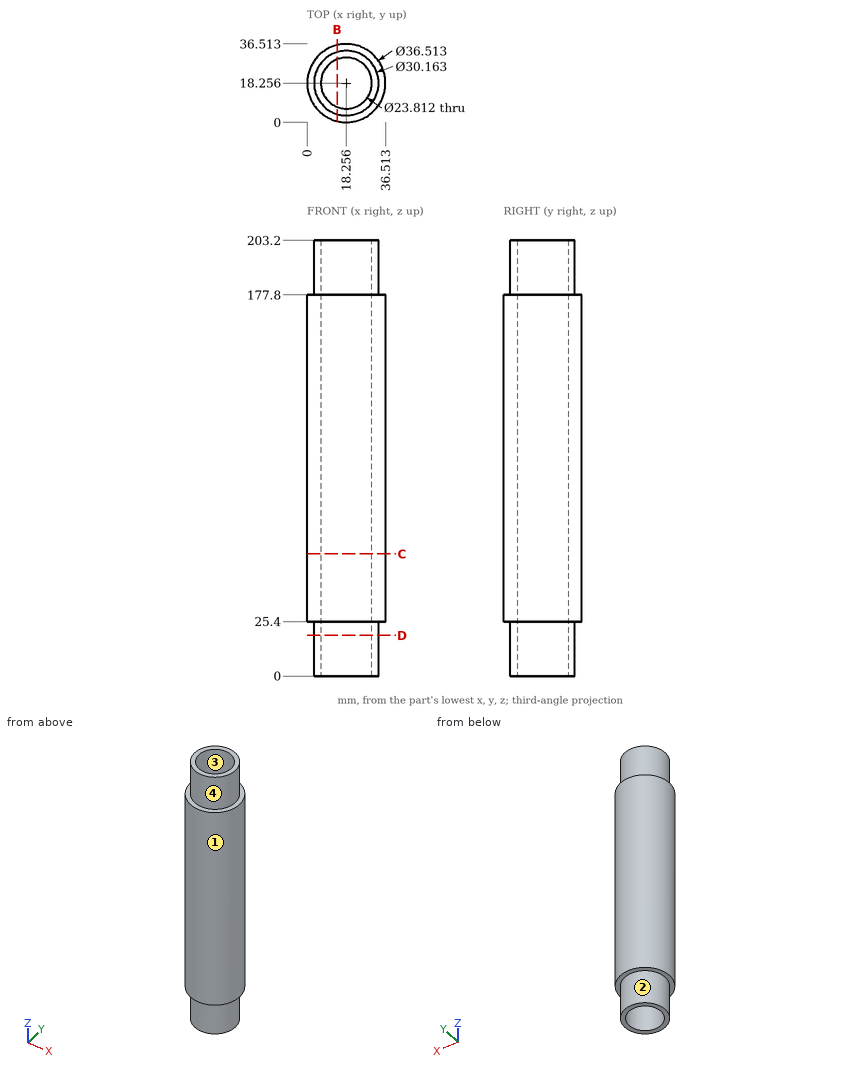
For this review, use the dimensioned drawing (mm, ordinates from the lowest corner) and the shaded views. A direction names the side the tool comes from. Round coordinates to 2 decimals unless told otherwise and drop trailing zeros. Write each loop counter-clockwise with the first axis right and the second up, starting at its lowest first coordinate (ties: lowest second). Pieces come first, ordered by that corner, then holes. Notation, with made-up numbers: (65.25, 21.25) -> (121.25, 21.25) arc R29 ccw to (121.25, 57.25) -> close; hole circle Ø11 at (56, 70.25). An arc over 180 degrees is marked (long way). Use one line per item in the form item = value.
Q1. Consider section C-C (z = 57). State the section outline as (x, y) points, then the cut area to 3 significant figures.
Resolved:
outline = circle Ø36.51 at (18.26, 18.26); hole circle Ø23.81 at (18.26, 18.26)
area = 602 mm²
Q2. To check wall thickness, follow probe 1 along X at (y, z) = (17.5, 181) (1 decimal); probe 2 along X at (y, z) = (18, 65); probe 3 along Z at (x, y) = (35, 12.5). State the ranges of each line that lie inside material, in increasing order. Write a range as from..to.
Resolved:
probe_1 = 3.2..6.4, 30.1..33.3
probe_2 = 0..6.35, 30.16..36.51
probe_3 = 25.4..177.8
Q3. Consider section D-D (z = 19). State the section outline as (x, y) points.
Resolved:
outline = circle Ø30.16 at (18.26, 18.26); hole circle Ø23.81 at (18.26, 18.26)
Q4. The part is to be moulded in two halves that separate along Y. For the marked faces 3 and 4, say which applies: released by +Y, released by -Y, zero draft, split by the parting line, or undercut.
Resolved:
face_3 = undercut
face_4 = split by the parting line
Q5. Clearance check with flat-ended pins moving along their axes: pin 1 Ø14.5 at (x, y) = (18.26, 18.26) entering from +Z; pin 2 Ø1.5 at (x, z) = (5, 101.5) entering from +Y (1 decimal); pin 3 Ø2 at (x, y) = (8.5, 4.5) entering from +Z; pin 4 Ø2 at (x, z) = (27, 145) entering from +Y. State where each tip first meets the part, or that it passes through.
Resolved:
pin_1 = through
pin_2 = 31.6
pin_3 = 177.8
pin_4 = 34.79
Q6. Machinability: for the marked faces 1 and 2, which of the approach directions +Z, -Z, +X, -X, +Y, -Y give a long, thin tool a straight path to every point of the face, cutting with its end or side? Answer none if there is none.
Resolved:
face_1 = +Z, -Z
face_2 = -Z
Q7. Consider section B-B (x = 14). State the section outline as (y, z) points (1 decimal), then the cut area to 3 significant figures.
Resolved:
outline = (0.5, 25.4) -> (3.8, 25.4) -> (3.8, 0) -> (7.1, 0) -> (7.1, 203.2) -> (3.8, 203.2) -> (3.8, 177.8) -> (0.5, 177.8) -> close; (29.4, 0) -> (32.7, 0) -> (32.7, 25.4) -> (36, 25.4) -> (36, 177.8) -> (32.7, 177.8) -> (32.7, 203.2) -> (29.4, 203.2) -> close
area = 2,360 mm²
